Part model, mm, in its own coordinate system. Face numbers are marked on the shaded views. A direction names the side the tool comes from. Coordinates: 2 decimals unless noted, no trailing zeros. Loops run counter-clockwise (first coordinate to the right, second up) from the corner with the lowest first, then second, coordinate; pieces in that order, holes last. Notation, with made-up numbers: (29.5, -7) - (81.5, -7) arc R11 ccw to (81.5, 7) - close; hole circle Ø10 at (-37, -18). An arc over 180 degrees is marked (long way). Use a Markdown table: item, result. Add a question column.
1. Band-saw the part on A-A, the plane z = 13.5. Give the cut face in (x, y).
2. 3-axis set-ups, long thin cutter, end or side, ignore diameter. For the marked faces 4 and 5: which of +Z, -Z, +X, -X, +Y, -Y reach the whole face in a straight line?
3. Band-saw the part on D-D, the plane x = -2. Give the cut face in (y, z), plus the area to 3 significant figures.
4. Wall check: probe 1 along Y at (x, z) = (-4.9, 17); probe 2 along X at (y, z) = (-1.25, 20.25); probe 3 along Z at (x, y) = (1.25, -0.75). Give the ranges that are in metal, low to high. Write a range as [from, to].
5. Band-saw the part on C-C, the plane y = 0.75. Give the cut face in (x, z), plus the area to 3 significant figures.
6. Pull direction X, two halves, no side cores. Call the marked faces 1, 2 and 3: pulls with the +X half, pulls with the -X half, needs draft (parallel to the pull), parting line crosses it, or undercut.
7. Drop flat-ended pins along their axis: pin 1 (3 mm diameter, centred on x = -1, y = 2, fed in from +Z); pin 2 (1 mm diameter, centred on x = -2, y = 3, fed in from +Z); pin 3 (2.5 mm diameter, centred on x = -0.5, y = 0, fed in from +Z). Give the stop position or say it passes through.
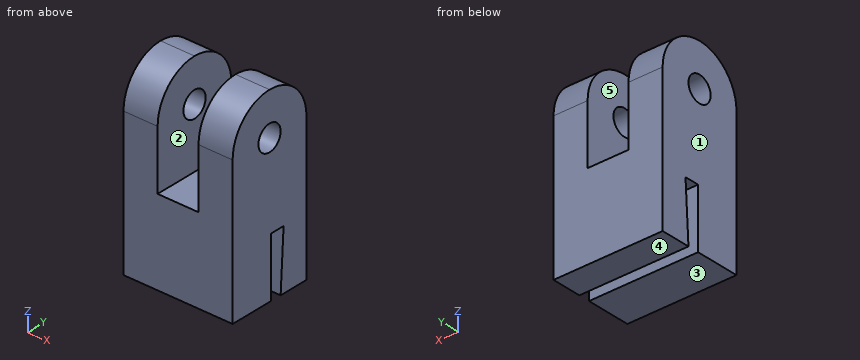
from build123d import *

# Parameters (mm, degrees)
BOSS_EXTRUDE1_DEPTH = 10
SKETCH1_3_W         = 12.8
SKETCH1_3_H         = 1.3
BOSS_EXTRUDE2_DEPTH = 7
SKETCH1_5_W         = 12.8
SKETCH1_5_H         = 1.3
CUT_EXTRUDE1_DEPTH  = 7
SKETCH4_W           = 12.8
SKETCH4_H           = 10
BOSS_EXTRUDE3_DEPTH = 1
CUT_EXTRUDE3_DEPTH  = 15
SKETCH8_W           = 12.8
SKETCH8_H           = 10
BOSS_EXTRUDE4_DEPTH = 1
SKETCH10_W          = 4
SKETCH10_H          = 10
BOSS_EXTRUDE5_DEPTH = 12
FILLET1_R           = 5
HOLE1_D             = 3
HOLE1_DEPTH         = 100


with BuildPart() as part:
    # Sketch1 → Boss-Extrude1 (new body)
    with BuildSketch(Plane.XY):
        Polygon((6.4, 4), (-6.4, 4), (-6.4, -1), (-6.4, -4), (6.4, -4), (6.4, -1), align=None)
    extrude(amount=BOSS_EXTRUDE1_DEPTH)

    # Sketch1<3> → Boss-Extrude2 (add)
    with BuildSketch(Plane.XY):
        with Locations((0, 1.85)):
            Rectangle(SKETCH1_3_W, SKETCH1_3_H)
    extrude(amount=BOSS_EXTRUDE2_DEPTH)

    # Sketch1<5> → Cut-Extrude1 (cut)
    with BuildSketch(Plane.XY):
        with Locations((0, 1.85)):
            Rectangle(SKETCH1_5_W, SKETCH1_5_H)
    extrude(amount=CUT_EXTRUDE1_DEPTH, mode=Mode.SUBTRACT)

    # Sketch4 → Boss-Extrude3 (add)
    with BuildSketch(Plane(origin=(0, 4, 0), x_dir=(1, 0, 0), z_dir=(0, 1, 0))):
        with Locations((0, -5)):
            Rectangle(SKETCH4_W, SKETCH4_H)
    extrude(amount=BOSS_EXTRUDE3_DEPTH)

    # Sketch6 → Cut-Extrude3 (cut)
    with BuildSketch(Plane(origin=(6.4, 0, 0), x_dir=(0, 0, -1), z_dir=(1, 0, 0))):
        Polygon((0, 2.5), (-7, 2.902751688), (-7, 2.5), align=None)
    extrude(amount=-CUT_EXTRUDE3_DEPTH, mode=Mode.SUBTRACT)

    # Sketch8 → Boss-Extrude4 (add)
    with BuildSketch(Plane(origin=(0, 5, 0), x_dir=(1, 0, 0), z_dir=(0, 1, 0))):
        with Locations((0, -5)):
            Rectangle(SKETCH8_W, SKETCH8_H)
    extrude(amount=BOSS_EXTRUDE4_DEPTH)

    # Sketch10 → Boss-Extrude5 (add)
    with BuildSketch(Plane.XY.offset(10)):
        with Locations((-4.4, 1)):
            Rectangle(SKETCH10_W, SKETCH10_H)
        with Locations((4.4, 1)):
            Rectangle(SKETCH10_W, SKETCH10_H)
    extrude(amount=BOSS_EXTRUDE5_DEPTH)

    # Fillet1
    fillet1_edges = [part.edges().sort_by_distance(p)[0] for p in [
        (-4.4, -4, 22),
        (-4.4, 6, 22),
        (4.4, -4, 22),
        (4.4, 6, 22),
    ]]
    fillet(fillet1_edges, radius=FILLET1_R - 0.0001)  # a hair under: the kernel refuses the full size

    # Hole1
    with Locations(Plane.ZY.offset(6.4)):
        with Locations((17, 1)):
            Hole(HOLE1_D / 2, depth=HOLE1_DEPTH)


solid = part.part
Geometry check:
| question | item | result |
|---|---|---|
| 1 | outline | (-6.4, -4) - (-2.4, -4) - (-2.4, 6) - (-6.4, 6) - close; (2.4, -4) - (6.4, -4) - (6.4, 6) - (2.4, 6) - close |
| 2 | face 4 | -Z, +X, -X, +Y, -Y |
| 2 | face 5 | +Z, +Y, -Y |
| 3 | outline | (-4, 0) - (1.2, 0) - (1.2, 7) - (2.9, 7) - (2.5, 0) - (6, 0) - (6, 10) - (-4, 10) - close |
| 3 | area | 89.5 mm^2 |
| 4 | probe 1 | y = [-4, -0.5], [2.5, 6] |
| 4 | probe 2 | x = [-6.4, -2.4], [2.4, 6.4] |
| 4 | probe 3 | z = [0, 10] |
| 5 | outline | (-6.4, 0) - (6.4, 0) - (6.4, 15.52) - (2.4, 15.52) - (2.4, 10) - (-2.4, 10) - (-2.4, 15.52) - (-6.4, 15.52) - close; (-6.4, 18.48) - (-2.4, 18.48) - (-2.4, 21.99) - (-6.4, 21.99) - close; (2.4, 18.48) - (6.4, 18.48) - (6.4, 21.99) - (2.4, 21.99) - close |
| 5 | area | 200 mm^2 |
| 6 | face 1 | pulls with the -X half |
| 6 | face 2 | undercut |
| 6 | face 3 | needs draft |
| 7 | pin 1 | stops at z = 21.98 |
| 7 | pin 2 | stops at z = 21.7 |
| 7 | pin 3 | stops at z = 10 |
